Work out the finished part from the listing and answer in its coordinate system (mm). A direction names the side the tool comes from. Give positions to 0.01 mm unless a question says otherwise; leave off trailing zeros. Order: outer loops, then holes, each group sorted by start corner. A loop starts at its lowest first (then second) coordinate and runs counter-clockwise, first axis right, second up. Notation, with made-up numbers: (-25, -1) - (-15, -1) arc R11 ccw to (-15, 15) - close; hole circle Ø10 at (83.25, 80.25). An arc over 180 degrees is marked (long way). Put each result on its own line as item: value.
```python
from build123d import *

# Parameters (mm, degrees)
SKETCH1_W                = 12.7
SKETCH1_H                = 14.2875
SKETCH1_R                = 1.5875
BOSS_EXTRUDE1_DEPTH      = 1.5875
SKETCH2_W                = 12.7
SKETCH2_H                = 3.175
BOSS_EXTRUDE2_DEPTH      = 1.5875
SKETCH3_R                = 0.396875
CUT_EXTRUDE1_DEPTH       = 5.7625
SKETCH4_R                = 0.396875
BOSS_EXTRUDE3_DEPTH      = 1.5875
BOSS_EXTRUDE3_DEPTH_BACK = 9.525
BOSS_EXTRUDE5_DEPTH      = 0.79375
BOSS_EXTRUDE5_DEPTH_BACK = 4.7625


with BuildPart() as part:
    # Sketch1 → Boss-Extrude1 (new body)
    with BuildSketch(Plane(origin=(0, 0, 0), x_dir=(1, 0, 0), z_dir=(0, 1, 0))):
        with Locations((6.35, -7.14375)):
            Rectangle(SKETCH1_W, SKETCH1_H)
        with Locations((10.16, -6.858)):
            Circle(SKETCH1_R, mode=Mode.SUBTRACT)
        with Locations((2.54, -6.858)):
            Circle(SKETCH1_R, mode=Mode.SUBTRACT)
    extrude(amount=-BOSS_EXTRUDE1_DEPTH)

    # Sketch2 → Boss-Extrude2 (add)
    with BuildSketch(Plane.XY.offset(14.2875)):
        with Locations((6.35, -3.175)):
            Rectangle(SKETCH2_W, SKETCH2_H)
    extrude(amount=-BOSS_EXTRUDE2_DEPTH)

    # Sketch3 → Cut-Extrude1 (cut, through all)
    with BuildSketch(Plane(origin=(0, 0, 0), x_dir=(1, 0, 0), z_dir=(0, 1, 0))):
        with Locations((0.79375, -13.49375)):
            Circle(SKETCH3_R)
        with Locations((3.58775, -13.49375)):
            Circle(SKETCH3_R)
        with Locations((6.38175, -13.49375)):
            Circle(SKETCH3_R)
        with Locations((9.17575, -13.49375)):
            Circle(SKETCH3_R)
        with Locations((11.96975, -13.49375)):
            Circle(SKETCH3_R)
    extrude(amount=-CUT_EXTRUDE1_DEPTH, mode=Mode.SUBTRACT)

    # Sketch4 → Boss-Extrude3 (add, two sides)
    with BuildSketch(Plane(origin=(0, 0, 0), x_dir=(1, 0, 0), z_dir=(0, 1, 0))) as boss_extrude3_sk:
        with Locations((0.79375, -13.49375)):
            Circle(SKETCH4_R)
        with Locations((3.58775, -13.49375)):
            Circle(SKETCH4_R)
        with Locations((6.38175, -13.49375)):
            Circle(SKETCH4_R)
        with Locations((9.17575, -13.49375)):
            Circle(SKETCH4_R)
        with Locations((11.96975, -13.49375)):
            Circle(SKETCH4_R)
    extrude(amount=BOSS_EXTRUDE3_DEPTH)
    extrude(boss_extrude3_sk.sketch, amount=-BOSS_EXTRUDE3_DEPTH_BACK)

    # Sketch5 → Boss-Extrude5 (add, two sides)
    with BuildSketch(Plane(origin=(0, 0, 0), x_dir=(-1, 0, 0), z_dir=(0, 0, -1))) as boss_extrude5_sk:
        with BuildLine():
            Line((-9.525, 0), (-10.062267539, 1.611802618))
            ThreePointArc((-10.062267539, 1.611802618), (-9.981921487, 2.138477744), (-9.507681244, 2.38125))
            Line((-9.507681244, 2.38125), (-3.065174491, 2.38125))
            ThreePointArc((-3.065174491, 2.38125), (-2.579253026, 2.12165746), (-2.524890791, 1.573430586))
            Line((-2.524890791, 1.573430586), (-3.175, 0))
            Line((-3.175, 0), (-9.525, 0))
        make_face()
    extrude(amount=BOSS_EXTRUDE5_DEPTH)
    extrude(boss_extrude5_sk.sketch, amount=-BOSS_EXTRUDE5_DEPTH_BACK)


solid = part.part
```
(1) Section A-A, the plane z = 4 is taken. Write down the section's boundary in (x, y) (1 decimal), then the cut area to 3 significant figures.
Geometry check:
outline: (0, -1.6) - (12.7, -1.6) - (12.7, 0) - (9.5, 0) - (10.1, 1.6) arc R0.6 ccw to (9.5, 2.4) - (3.1, 2.4) arc R0.6 ccw to (2.5, 1.6) - (3.2, 0) - (0, 0) - close
area: 37.1 mm²
(2) A tool of negligible diameter and unlimited length cuts with its end or side. For faces 4 (the face through (6, -2, 14.288)), 5 (the face through (6, -3, 12.7)), 6 (the face through (2.845, 0.798, 1.945)), 7 (the face through (6, -4.762, 14)), from which of +Z, -Z, +X, -X, +Y, -Y can it reach the whole face along a straight path? Write none if from no direction.
Geometry check:
face 4: +Z, +X, -X, +Y, -Y
face 5: -Z, +X, -X, -Y
face 6: +Z, -Z, -X
face 7: -Y
(3) Section B-B, the plane x = 1.75 is taken. Write down the section's boundary in (y, z).
Geometry check:
outline: (-4.76, 12.7) - (-1.59, 12.7) - (-1.59, 8.23) - (0, 8.23) - (0, 14.29) - (-4.76, 14.29) - close; (-1.59, 0) - (0, 0) - (0, 5.48) - (-1.59, 5.48) - close
(4) Section D-D, the plane y = -6.75 is taken. Write down the section's boundary in (x, z), then the cut area to 3 significant figures.
Geometry check:
outline: circle Ø0.79 at (0.79, 13.49); circle Ø0.79 at (3.59, 13.49); circle Ø0.79 at (6.38, 13.49); circle Ø0.79 at (9.18, 13.49); circle Ø0.79 at (11.97, 13.49)
area: 2.47 mm²
(5) Determine the mould class of faces 1 (the face through (6, 1, 4.762)), 2 (the face through (9.79, 0.79, 1.95)), 3 (the face through (6, -1.588, 6)) for opening direction Y: pulls with the +Y half, pulls with the -Y half, needs draft (parallel to the pull), parting line crosses it, or undercut.
Geometry check:
face 1: needs draft
face 2: undercut
face 3: pulls with the -Y half
(6) Section C-C, the plane x = 4.5 is taken. Write down the section's boundary in (y, z), then the cut area to 3 significant figures.
Geometry check:
outline: (-4.76, 12.7) - (-1.59, 12.7) - (-1.59, 0) - (0, 0) - (0, -0.79) - (2.38, -0.79) - (2.38, 4.76) - (0, 4.76) - (0, 14.29) - (-4.76, 14.29) - close
area: 41.0 mm²
(7) Given pin 1 (2.5 mm diameter, centred on x = 7, y = -2.5, fed in from -Z); pin 2 (3 mm diameter, centred on x = 9.5, z = 2, fed in from -Y); pin 3 (1.2 mm diameter, centred on x = 5, y = 1.5, fed in from +Z); pin 4 (1.3 mm diameter, centred on x = 4, z = 14, fed in from -Y) (3 decimals), each flat-ended and moving along its own axis, determine where each tip first touches the part or whether it passes through.
Geometry check:
pin 1: stops at z = 0
pin 2: stops at y = -1.59
pin 3: stops at z = 4.76
pin 4: stops at y = -9.525
(8) Straight lines are drawn through the part: line 1 (Z direction, x = 10.16, y = -1.1); line 2 (Y direction, x = 9.5, z = 9.5); line 3 (Y direction, x = 2.75, z = 13.5). For each, find the intervals that lie inside material, in ascending order.
Geometry check:
line 1: z = 0 to 5.27, 8.45 to 14.29
line 2: y = -1.59 to 0
line 3: y = -4.76 to 0
